For this review, take the finished solid that the model builds, in its own axes (mm). Give positions to 0.01 mm unless a question says otherwise; leave off trailing zeros. Order: outer loops, then holes, each group sorted by start corner. A loop starts at its lowest first (then second) coordinate and runs counter-clockwise, first axis right, second up. Notation, with made-up numbers: (-16.75, -36.5) - (13.25, -36.5) arc R36 ccw to (13.25, -0.5) - close; hole circle Ø9 at (72, -3). An arc over 180 degrees is marked (long way). One line per item, written item: value.
Autodesk Inventor part; units mm, degrees
ref_plane "YZ Plane" through (0, 0, 0) normal (1, 0, 0) x (0, 1, 0)
ref_plane "XZ Plane" through (0, 0, 0) normal (0, 1, 0) x (-1, 0, 0)
ref_plane "XY Plane" through (0, 0, 0) normal (0, 0, 1) x (1, 0, 0)
sketch "Sketch1" plane through (0, 0, 0) normal (0, 0, 1) x (1, 0, 0)
  line L0 (48, -210) -> (48, -398)
  arc A0 (46, -400) -> (48, -398) centre (46, -398) ccw
  line L1 (46, -400) -> (-14, -400)
  line L2 (-16, -398) -> (-16, -210)
  arc A1 (-16, -398) -> (-14, -400) centre (-14, -398) ccw
  line L3 (48, -114.5) -> (48, -269.5)
  line L4 (48, 14) -> (48, -174)
  line L5 (-16, -174) -> (-16, 14)
  line L6 (-14, 16) -> (46, 16)
  arc A2 (-14, 16) -> (-16, 14) centre (-14, 14) ccw
  arc A3 (48, 14) -> (46, 16) centre (46, 14) ccw
  circle A4 centre (32, -184) radius 1.85
  circle A5 centre (37.6569, -186.3431) radius 1.85
  circle A6 centre (40, -192) radius 1.85
  circle A7 centre (32, -192) radius 4
  circle A8 centre (37.6569, -197.6569) radius 1.85
  circle A9 centre (24, -192) radius 1.85
  circle A10 centre (26.3431, -186.3431) radius 1.85
  circle A11 centre (26.3431, -197.6569) radius 1.85
  circle A12 centre (32, -200) radius 1.85
  circle A13 centre (37.6569, -101.6569) radius 1.85
  circle A14 centre (40, -96) radius 1.85
  circle A15 centre (37.6569, -90.3431) radius 1.85
  circle A16 centre (32, -88) radius 1.85
  circle A17 centre (32, -96) radius 4
  circle A18 centre (26.3431, -90.3431) radius 1.85
  circle A19 centre (24, -96) radius 1.85
  circle A20 centre (26.3431, -101.6569) radius 1.85
  circle A21 centre (32, -104) radius 1.85
  circle A22 centre (24, -288.0038) radius 1.85
  circle A23 centre (26.3431, -293.6606) radius 1.85
  circle A24 centre (32, -296.0038) radius 1.85
  circle A25 centre (37.6569, -293.6606) radius 1.85
  circle A26 centre (40, -288.0038) radius 1.85
  circle A27 centre (37.6569, -282.3469) radius 1.85
  circle A28 centre (32, -280.0038) radius 1.85
  circle A29 centre (26.3431, -282.3469) radius 1.85
  circle A30 centre (32, -288.0038) radius 4
  circle A31 centre (24, -264) radius 1.85
  circle A32 centre (24, -216) radius 1.85
  circle A33 centre (24, -168) radius 1.85
  circle A34 centre (24, -120) radius 1.85
  line L7 (-16, -210) -> (-16, -174)
  circle A35 centre (32, -352) radius 3.925
  circle A36 centre (32, -32) radius 3.925
  point P0 (0, 0)
  point P1 (16, -176)
  point P2 (16, -208)
extrude "Extrusion1" add sketch "Sketch1" along normal blind 2
sketch "Sketch3" plane through (0, 0, 2) normal (0, 0, 1) x (1, 0, 0)
  arc A0 (17, -162.5) -> (17, -125.5) centre (17, -144) ccw
  arc A1 (17, -258.5) -> (17, -221.5) centre (17, -240) ccw
  circle A2 centre (17, -144) radius 18.5
  circle A3 centre (17, -240) radius 18.5
  point P0 (0, 0)
  point P1 (17, -221.5)
  point P2 (17, -125.5)
extrude "Extrusion3" cut sketch "Sketch3" against normal through all
sketch "Sketch4" plane through (0, 0, 2) normal (0, 0, 1) x (1, 0, 0)
  circle A0 centre (17, -144) radius 18.65
  circle A1 centre (17, -240) radius 18.65
  arc A2 (8, -120.2479) -> (-8.4, -144) centre (17, -144) ccw
  arc A3 (-8.4, -240) -> (8, -263.7521) centre (17, -240) ccw
  line L0 (8, -263.7521) -> (8, -400)
  line L1 (8, 16) -> (8, -120.2479)
  line L2 (8, -400) -> (-14, -400)
  line L3 (8, 16) -> (-14, 16)
  arc A4 (-14, 16) -> (-16, 14) centre (-14, 14) ccw
  arc A5 (-16, -398) -> (-14, -400) centre (-14, -398) ccw
  line L4 (-8.4, -240) -> (-8.4, -208)
  line L5 (-8.4, -176) -> (-8.4, -144)
  line L6 (-16, 14) -> (-16, -398)
  line L7 (-16, -398) -> (-16, 14)
  line L8 (-8.4, -208) -> (-8.4, -176)
  point P0 (0, 0)
  dimension "d8" = 50.8
extrude "Extrusion4" cut sketch "Sketch4" against normal through all contours A2 L5 L8 L4 A3 L0 L2 A5 L6 A4 L3 L1
sketch "Sketch5" plane through (0, 0, 0) normal (0, 0, -1) x (-1, 0, 0)
  line L0 (-48, -96) -> (-46, -96)
  line L1 (-46, -288) -> (-48, -288)
  line L2 (-46, -288) -> (-46, -96)
  line L3 (-48, -398) -> (-48, 14)
  line L4 (-48, -96) -> (-48, -288)
  point P0 (0, 0)
extrude "Extrusion5" cut sketch "Sketch5" against normal through all
sketch "Sketch6" plane through (0, 0, 2) normal (0, 0, 1) x (1, 0, 0)
  circle A0 centre (40, 6.4) radius 1.85
  circle A1 centre (24, 6.4) radius 1.85
  circle A2 centre (40, -390.4) radius 1.85
  circle A3 centre (24, -390.4) radius 1.85
  point P0 (0, 0)
extrude "Extrusion6" cut sketch "Sketch6" against normal through all
properties part number "plate1" material "Aluminum 6061"
(1) Draft analysis for pull direction X (two halves, no side actions). For faces 1 (the face through (31.49, -355.89, 0.99)), 2 (the face through (26, -189, 0)), 3 (the face through (-4.023, -254.255, 1.014)), state which applies: pulls with the +X half, pulls with the -X half, needs draft (parallel to the pull), parting line crosses it, or undercut.
Answers below:
face 1: undercut
face 2: needs draft
face 3: pulls with the -X half
(2) Take a section at A-A (y = -352). Write out the cut boundary in (x, z) (3 decimals).
Answers below:
outline: (8, 0) - (28.075, 0) - (28.075, 2) - (8, 2) - close; (35.925, 0) - (48, 0) - (48, 2) - (35.925, 2) - close
(3) Wall thickness on line 1 (X direction, y = -186, z = 0.85); line 2 (Y direction, x = 40, z = 0.8); line 3 (Y direction, x = 19, z = 1.3): over which ranges is each line inside the solid? List them lowest first. Write a range as from..to.
Answers below:
line 1: x = -8.4..24.53, 28.16..35.84, 39.47..46
line 2: y = -400..-392.25, -388.55..-289.85, -286.15..-193.85, -190.15..-97.85, -94.15..4.55, 8.25..16
line 3: y = -400..-258.39, -221.61..-162.39, -125.61..16
(4) For P1, Ø1, axis at y = -48.5, z = 0.5, coming from the -X side; P2, Ø1, axis at y = -168, z = 2, coming from the +X side; P3, Ø1, axis at x = -1, z = 1.5, coming from the -Y side, all flat-tipped, find the tip position at first contact; note any pin that passes through.
Answers below:
P1: stops at x = 8
P2: stops at x = 46
P3: stops at y = -258.41
(5) Take a section at D-D (z = 1.55). Give the number of separate pieces and of enclosed holes in the cut face, then the cut area to 3 significant figures.
Answers below:
separate pieces: 1
enclosed holes: 39
area: 15,700 mm^2
(6) Take a section at B-B (x = 17). Write out the cut boundary in (y, z).
Answers below:
outline: (-400, 0) - (-258.5, 0) - (-258.5, 2) - (-400, 2) - close; (-221.5, 0) - (-162.5, 0) - (-162.5, 2) - (-221.5, 2) - close; (-125.5, 0) - (16, 0) - (16, 2) - (-125.5, 2) - close
(7) Take a section at C-C (y = -129.5). Write out the cut boundary in (x, z).
Answers below:
outline: (-3.85, 0) - (5.51, 0) - (5.51, 2) - (-3.85, 2) - close; (28.49, 0) - (46, 0) - (46, 2) - (28.49, 2) - close
